Model file for the job. Use its own axes, mm. A direction names the side the tool comes from. Give positions to 0.01 mm unless a question says otherwise; leave off trailing zeros. Write each loop counter-clockwise with the first axis right and the second up, starting at its lowest first coordinate (ties: lowest second). Pieces come first, ordered by that corner, then holes. Notation, with made-up numbers: (-12.5, 71.5) - (46.5, 71.5) arc R20 cw to (46.5, 93.5) - close; hole circle Ø2 at (1, 78). An arc over 180 degrees is marked (long way). One line per item, written item: value. Start each with the question number.
(1) Cut at B-B, the plane y = 52.5. List the corners of the cut face in (x, z).
(2) Probe L1, parallel to Y at x = 18, z = -46.5; L2, parallel to Z at x = 0, y = 55.25; L3, parallel to Z at x = -9, y = 10.5. List the from-to ranges inside material, lowest first.
(3) Cut at A-A, the plane x = 0. List the corners of the cut face in (y, z), and give its area (3 significant figures).
(4) Cut at D-D, the plane z = -11.5. List the corners of the cut face in (x, y).
(5) Mould opens along X. For faces 1 (the face through (25.96, -52.4, -58.49)), 2 (the face through (0.603, 14.988, -14.79)), 3 (the face through (0, 60, -53)) say: pulls with the +X half, pulls with the -X half, needs draft (parallel to the pull), parting line crosses it, or undercut.
(6) Cut at C-C, the plane z = -65. List the corners of the cut face in (x, y).
(7) Drop flat-ended pins along their axis: P1, Ø4, axis at x = -0.5, z = -16.5, coming from the +Y side; P2, Ø9.5, axis at x = 0, z = -65, coming from the -Y side; P3, Ø4, axis at y = -17, z = -9.5, coming from the -X side; P4, Ø18, axis at x = -6, y = -24.5, coming from the +Z side. Give the stop position or say it passes through.
(8) 3-axis set-ups, long thin cutter, end or side, ignore diameter. For faces 4 (the face through (-6, -45, -57)), 5 (the face through (-29.97, 1.32, -14.79)), 6 (the face through (0, 43, -30)): which of +Z, -Z, +X, -X, +Y, -Y reach the whole face in a straight line?
from build123d import *

# Parameters (mm, degrees)
SKETCH1_R           = 30
BOSS_EXTRUDE1_DEPTH = 30
SKETCH2_W           = 60
SKETCH2_H           = 90
BOSS_EXTRUDE2_DEPTH = 15
SKETCH3_R           = 8
BOSS_EXTRUDE3_DEPTH = 15


with BuildPart() as part:
    # Sketch1 → Boss-Extrude1 (new body)
    with BuildSketch(Plane.XY):
        Circle(SKETCH1_R)
        with BuildLine():
            Line((-4, -14.456832295), (-4, -17.956832295))
            Line((-4, -17.956832295), (4, -17.956832295))
            Line((4, -17.956832295), (4, -14.456832295))
            ThreePointArc((4, -14.456832295), (0, 15), (-4, -14.456832295))
        make_face(mode=Mode.SUBTRACT)
    extrude(amount=-BOSS_EXTRUDE1_DEPTH)

    # Sketch2 → Boss-Extrude2 (add)
    with BuildSketch(Plane(origin=(0, 0, -30), x_dir=(-1, 0, 0), z_dir=(0, 0, -1))):
        Rectangle(SKETCH2_W, SKETCH2_H)
    extrude(amount=BOSS_EXTRUDE2_DEPTH)

    # Sketch3 → Boss-Extrude3 (add)
    with BuildSketch(Plane(origin=(0, 45, 0), x_dir=(1, 0, 0), z_dir=(0, 1, 0))):
        with BuildLine():
            Line((-30, 45), (-22.03289839, 71.599347585))
            ThreePointArc((-22.03289839, 71.599347585), (0, 88), (22.03289839, 71.599347585))
            Line((22.03289839, 71.599347585), (30, 45))
            Line((30, 45), (30, 30))
            Line((30, 30), (-30, 30))
            Line((-30, 30), (-30, 45))
        make_face()
        with Locations(Location((0, 65, 0), (0, 0, 180))):
            Circle(SKETCH3_R, mode=Mode.SUBTRACT)
    boss_extrude3 = extrude(amount=BOSS_EXTRUDE3_DEPTH)

    # Mirror1: Boss-Extrude3 across plane
    add(boss_extrude3.mirror(Plane.ZX))


solid = part.part
Answers follow:
1. outline: (-30, -45) - (-22.03, -71.6) arc R23 ccw to (22.03, -71.6) - (30, -45) - (30, -30) - (-30, -30) - close; hole circle Ø16 at (0, -65)
2. L1: y = -60 to -45, 45 to 60
2. L2: z = -88 to -73, -57 to -30
2. L3: z = -45 to -30
3. outline: (-60, -88) - (-45, -88) - (-45, -73) - (-60, -73) - close; (-60, -57) - (-45, -57) - (-45, -45) - (45, -45) - (45, -57) - (60, -57) - (60, -30) - (30, -30) - (30, 0) - (15, 0) - (15, -30) - (-17.96, -30) - (-17.96, 0) - (-30, 0) - (-30, -30) - (-60, -30) - close; (45, -88) - (60, -88) - (60, -73) - (45, -73) - close
3. area: 3,420 mm²
4. outline: circle Ø60 at (0, 0); hole (-4, -17.96) - (4, -17.96) - (4, -14.46) arc R15 ccw (long way) to (-4, -14.46) - close
5. face 1: pulls with the +X half
5. face 2: undercut
5. face 3: needs draft
6. outline: (-24.01, -60) - (-8, -60) - (-8, -45) - (-24.01, -45) - close; (-24.01, 45) - (-8, 45) - (-8, 60) - (-24.01, 60) - close; (8, -60) - (24.01, -60) - (24.01, -45) - (8, -45) - close; (8, 45) - (24.01, 45) - (24.01, 60) - (8, 60) - close
7. P1: stops at y = 30
7. P2: passes through
7. P3: stops at x = -25.98
7. P4: stops at z = 0
8. face 4: -Z, +X, -X
8. face 5: +Z
8. face 6: +Z, +Y
